The listing builds one solid part. Answer for the finished solid, in the listing's coordinates (mm). A direction names the side the tool comes from. Coordinates: 2 decimals unless noted, no trailing zeros. Write each loop counter-clockwise with the first axis right and the second up, starting at its lowest first coordinate (ties: lowest second). Pieces come first, ordered by that corner, then holes. Notation, with made-up numbers: M 78.25,49.25 L 116.25,49.25 A8 cw 116.25,64.25 Z; hole C 84,-22 d3. An arc over 180 degrees is marked long. Answer as a JSON object with one key per item and string values. Group by question number.
from build123d import *

# Parameters (mm, degrees)
SZKIC1_R                    = 72.5
SZKIC1_R_2                  = 2
SZKIC1_R_3                  = 55
DODANIE_WYCI_GNI_CIE1_DEPTH = 4
SZKIC1_3_R                  = 72.5
SZKIC1_3_R_2                = 68.5
SZKIC1_3_R_3                = 59
SZKIC1_3_R_4                = 55
DODANIE_WYCI_GNI_CIE2_DEPTH = 34
DODANIE_WYCI_GNI_CIE3_DEPTH = 30
SZYK_KO_OWY1_COUNT          = 10


with BuildPart() as part:
    # Szkic1 → Dodanie-wyci_gni_cie1 (new body)
    with BuildSketch(Plane.XY):
        Circle(SZKIC1_R)
        with Locations((19.699833391, 60.629852914)):
            Circle(SZKIC1_R_2, mode=Mode.SUBTRACT)
        with Locations((63.75, 0)):
            Circle(SZKIC1_R_2, mode=Mode.SUBTRACT)
        with Locations((19.699833391, -60.629852914)):
            Circle(SZKIC1_R_2, mode=Mode.SUBTRACT)
        with Locations((-51.574833391, -37.471309834)):
            Circle(SZKIC1_R_2, mode=Mode.SUBTRACT)
        with Locations((-51.574833391, 37.471309834)):
            Circle(SZKIC1_R_2, mode=Mode.SUBTRACT)
        Circle(SZKIC1_R_3, mode=Mode.SUBTRACT)
    extrude(amount=DODANIE_WYCI_GNI_CIE1_DEPTH)

    # Szkic1_3 → Dodanie-wyci_gni_cie2 (add)
    # profile 1 of 2: a face of its own
    with BuildSketch(Plane.XY):
        Circle(SZKIC1_3_R)
        Circle(SZKIC1_3_R_2, mode=Mode.SUBTRACT)
    # profile 2 of 2: a face of its own
    with BuildSketch(Plane.XY):
        Circle(SZKIC1_3_R_3)
        Circle(SZKIC1_3_R_4, mode=Mode.SUBTRACT)
    extrude(amount=DODANIE_WYCI_GNI_CIE2_DEPTH)

    # Szkic2 → Dodanie-wyci_gni_cie3 (add)
    with BuildSketch(Plane.XY.offset(4)):
        Polygon((-2.5, 58.947010102), (-2.5, 68.45436436), (0, 72.265754907), (2.5, 68.45436436), (2.5, 58.947010102), (0, 55.135619556), align=None)
    dodanie_wyci_gni_cie3 = extrude(amount=DODANIE_WYCI_GNI_CIE3_DEPTH)

    # Szyk ko_owy1: Dodanie-wyci_gni_cie3 ×10 about axis
    szyk_ko_owy1_axis = Axis((0, 0, 0), (0, 0, 1))
    for i in range(1, SZYK_KO_OWY1_COUNT):
        add(dodanie_wyci_gni_cie3.rotate(szyk_ko_owy1_axis, i * 360 / SZYK_KO_OWY1_COUNT))


solid = part.part
Item 1: A cutting plane is placed at A-A, the plane y = 0. Write down the section's boundary in (x, z).
Item 2: For a pull along Y with two mould halves and no side action, classify faces 1 (the face through (69.15, 21.78, 16.76)), 2 (the face through (-21, 59, 4)) as +Y half, -Y half, draft (parallel to the pull), parting line (faces both ways), or undercut.
Item 3: A cutting plane is placed at C-C, the plane z = 24. State how many separate pieces and enclosed holes the cut face has, and give its area (3 significant figures).
Item 4: Flat-ended cylindrical pins translate along their axes: pin 1 Ø5 at (x, z) = (39, 22.5) entering from -Y; pin 2 Ø5 at (y, z) = (64.5, 16) entering from -X; pin 3 Ø1.5 at (y, z) = (50, 7.5) entering from +X; pin 4 Ø3 at (x, y) = (-51.57, 37.47) entering from +Z. Find the tip coordinate at first contact, or state that the pin passes through.
Item 5: A cutting plane is placed at D-D, the plane x = -18.5. Write down the section's boundary in (y, z), and give its area (3 significant figures).
Item 6: A cutting plane is placed at B-B, the plane x = 0. Write down the section's boundary in (y, z), and give its area (3 significant figures).
Item 7: A tool of negligible diameter and unlimited length cuts with its end or side. For faces 3 (the face through (61.752, 0.088, 1.972)), 4 (the face through (-59.87, 22.08, 18.79)), from which of +Z, -Z, +X, -X, +Y, -Y can it reach the whole face along a straight path? Write none if from no direction.
Item 8: Consider L1, parallel to X at y = -2, z = 26; L2, parallel to Y at x = 0, z = 21; L3, parallel to Y at x = -35.5, z = 16. Determine where each line is inside the solid, lowest interval first. Write a range as from..to.
Answer:
{
 "1": {"outline": "M -72.5,0 L -55,0 L -55,34 L -59,34 L -59,4 L -68.5,4 L -68.5,34 L -72.5,34 Z; M 55,0 L 61.75,0 L 61.75,4 L 59,4 L 59,34 L 55,34 Z; M 65.75,0 L 72.5,0 L 72.5,34 L 68.5,34 L 68.5,4 L 65.75,4 Z"},
 "2": {"face 1": "parting line", "face 2": "undercut"},
 "3": {"separate pieces": "1", "enclosed holes": "11", "area": "3,680 mm2"},
 "4": {"pin 1": "y = -62.64", "pin 2": "x = -37.58", "pin 3": "x = 53.2", "pin 4": "through"},
 "5": {"outline": "M -70.1,0 L -51.8,0 L -51.8,34 L -56.02,34 L -56.02,4 L -65.95,4 L -65.95,34 L -70.1,34 Z; M 51.8,0 L 70.1,0 L 70.1,34 L 65.95,34 L 65.95,4 L 56.02,4 L 56.02,34 L 51.8,34 Z", "area": "649 mm2"},
 "6": {"outline": "M -72.5,0 L -55,0 L -55,34 L -72.5,34 Z; M 55,0 L 72.5,0 L 72.5,34 L 55,34 Z", "area": "1,190 mm2"},
 "7": {"face 3": "+Z, -Z", "face 4": "+Z"},
 "8": {"L1": "-72.47..-68.47, -58.97..-54.96, 54.96..58.97, 68.47..72.47", "L2": "-72.5..-55, 55..72.5", "L3": "-63.21..-58.58, -53.11..-42.01, 42.01..53.11, 58.58..63.21"}
}
